from build123d import *

# Parameters (mm, degrees)
F1_DEPTH = 2
F0_W     = 30
F0_H     = 50
F2_DEPTH = 3
F3_DEPTH = 4


with BuildPart() as f1:
    # F0 (on Top) → F1 (new body)
    with BuildSketch(Plane.XY):
        Polygon((-17.329822, 20.581069), (-47.329822, 20.581069), (-47.329822, -29.418931), (-47.329822, -99.418931), (-42.329822, -109.418931), (-37.329822, -99.418931), (-37.329822, -29.418931), (-17.329822, -29.418931), align=None)
    extrude(amount=-F1_DEPTH)

    # F0 (on Top) → F2 (join)
    with BuildSketch(Plane.XY):
        with Locations((-2.329822, -4.418931)):
            Rectangle(F0_W, F0_H)
    extrude(amount=-F2_DEPTH)

    # F0 (on Top) → F3 (join)
    with BuildSketch(Plane.XY):
        with Locations((27.670178, -4.418931)):
            Rectangle(F0_W, F0_H)
    extrude(amount=-F3_DEPTH)


solid = f1.part
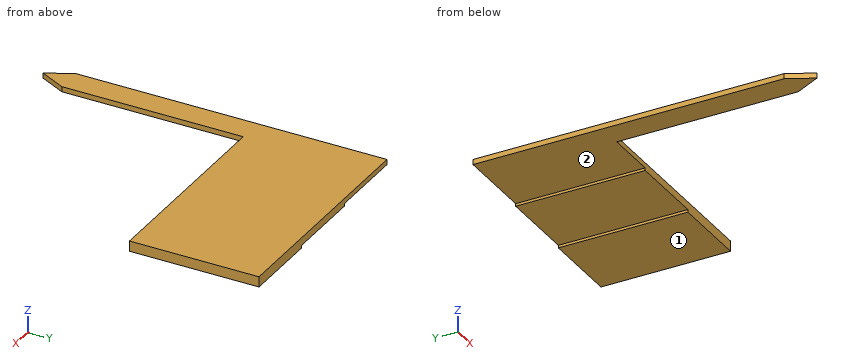
Here's how the part is built. I have some questions about the finished solid (model axes, mm). Face numbers are marked on the shaded views. A direction names the side the tool comes from. Give positions to 0.01 mm unless a question says otherwise; leave off trailing zeros. Loops run counter-clockwise (first coordinate to the right, second up) from the corner with the lowest first, then second, coordinate; pieces in that order, holes last. Notation, with made-up numbers: (73.5, -4.75) -> (103.5, -4.75) arc R7 ccw to (103.5, 0.25) -> close; hole circle Ø8 at (-6.5, -4.75). An arc over 180 degrees is marked (long way). One line per item, written item: value.
Q1. Suppose I cut it at A-A on y = -9.5. Please give me the cut outline in (x, z).
Answers follow:
outline: (-47.33, -2) -> (-17.33, -2) -> (-17.33, -3) -> (12.67, -3) -> (12.67, -4) -> (42.67, -4) -> (42.67, 0) -> (-47.33, 0) -> close
Q2. On a 3-axis mill with a long thin cutter (end or side, diameter ignored), from which of +Z, -Z, +X, -X, +Y, -Y can I reach the whole of each face in a straight line? I mean the marked faces 1 and 2. Say none if no direction works.
Answers follow:
face 1: -Z, +X, -X, +Y, -Y
face 2: -Z, -X, +Y, -Y
Q3. Suppose I cut it at D-D on y = -60. Please give me the cut outline in (x, z), then the cut area to 3 significant figures.
Answers follow:
outline: (-47.33, -2) -> (-37.33, -2) -> (-37.33, 0) -> (-47.33, 0) -> close
area: 20.0 mm^2
Q4. If I drill on line 1 along Z through (x, y) = (-19.5, 10.5); line 2 along X through (y, z) = (-35, -0.4); line 3 along Y through (x, z) = (39.5, -1.3), over which ranges is the centre line in solid material (lowest first)?
Answers follow:
line 1: -2 to 0
line 2: -47.33 to -37.33
line 3: -29.42 to 20.58
Q5. Suppose I cut it at B-B on z = -1. Please give me the cut outline in (x, y), then the cut area to 3 significant figures.
Answers follow:
outline: (-47.33, -99.42) -> (-42.33, -109.42) -> (-37.33, -99.42) -> (-37.33, -29.42) -> (42.67, -29.42) -> (42.67, 20.58) -> (-47.33, 20.58) -> close
area: 5,250 mm^2
Q6. Suppose I cut it at C-C on x = -9. Please give me the cut outline in (y, z), then the cut area to 3 significant figures.
Answers follow:
outline: (-29.42, -3) -> (20.58, -3) -> (20.58, 0) -> (-29.42, 0) -> close
area: 150 mm^2
Q7. I'm going to push flat-ended pins straight in: pin 1 Ø0.8 at (y, z) = (3.5, -2.5) entering from -X; pin 2 Ø9 at (x, y) = (-0.5, -8.5) entering from -Z; pin 3 Ø1.6 at (y, z) = (-64, -1) entering from +X. Where does each tip first touch, or does it pass through?
Answers follow:
pin 1: x = -17.33
pin 2: z = -3
pin 3: x = -37.33
